Autodesk Inventor part; units mm, degrees
ref_plane "YZ Plane" through (0, 0, 0) normal (1, 0, 0) x (0, 1, 0)
ref_plane "XZ Plane" through (0, 0, 0) normal (0, 1, 0) x (-1, 0, 0)
ref_plane "XY Plane" through (0, 0, 0) normal (0, 0, 1) x (1, 0, 0)
sketch "スケッチ1" plane through (0, 0, 0) normal (0, 0, 1) x (1, 0, 0)
  line L0 (0, 0) -> (122, 0)
  line L1 (122, 0) -> (122, 22)
  line L2 (122, 22) -> (0, 22)
  line L3 (0, 22) -> (0, 0)
  dimension "d0" = 122
  dimension "d1" = 22
extrude "押し出し1" add sketch "スケッチ1" along normal blind 2
fillet "フィレット1" radius 2 4 edges at (122, 22, 1) (122, 0, 1) (0, 22, 1) (0, 0, 1)
sketch "スケッチ2" plane through (0, 0, 2) normal (0, 0, 1) x (1, 0, 0)
  line L0 (0, 4.5) -> (122, 4.5)
  line L1 (122, 2) -> (122, 20)
  line L2 (2, 0) -> (120, 0)
  line L3 (0, 20) -> (0, 2)
  point P0 (0, 0)
  point P1 (11, 4.5)
  point P2 (31, 4.5)
  point P3 (51, 4.5)
  point P4 (61, 4.5)
  point P5 (71, 4.5)
  point P6 (91, 4.5)
  point P7 (111, 4.5)
  dimension "d5" = 4.5
  dimension "d6" = 11
  dimension "d7" = 11
  dimension "d8" = 20
  dimension "d9" = 20
  dimension "d10" = 10
  dimension "d11" = 10
  dimension "d12" = 20
hole "穴1" at (11, 4.5, 2) at (31, 4.5, 2) at (51, 4.5, 2) at (61, 4.5, 2) at (71, 4.5, 2) at (91, 4.5, 2) at (111, 4.5, 2) direction (0, 0, -1) diameter 3.2 end through all
properties part number "line_sensor" material "アセタール樹脂、黒"
Read the model definition and answer for the solid it produces. Units are mm, in the model's axes. Round coordinates to 2 decimals unless told otherwise and drop trailing zeros. Write each loop counter-clockwise with the first axis right and the second up, starting at its lowest first coordinate (ties: lowest second). Pieces come first, ordered by that corner, then holes.
Q1. A straight line is drawn through the part: line 1 (Y direction, x = 51, z = 1.45). Find the intervals that lie inside material, in ascending order.
Values:
line 1: y = 0 to 2.9, 6.1 to 22
Q2. Find section C-C on y = 4.5. State how many separate pieces and enclosed holes the cut face has, and give its area (3 significant figures).
Values:
separate pieces: 8
enclosed holes: 0
area: 199 mm2
Q3. The mould has two halves that part along X. Classify faces 1 (the face through (0, 11, 1)), 2 (the face through (121.4, 0.57, 1.01)), 3 (the face through (89.414, 4.708, 0.986)), 4 (the face through (60, 0, 1)): released by +X, released by -X, zero draft, split by the parting line, or undercut.
Values:
face 1: released by -X
face 2: released by +X
face 3: undercut
face 4: zero draft
Q4. Find section B-B on z = 1.3. Determine the outline of the cut face in (x, y).
Values:
outline: (0, 2) arc R2 ccw to (2, 0) - (120, 0) arc R2 ccw to (122, 2) - (122, 20) arc R2 ccw to (120, 22) - (2, 22) arc R2 ccw to (0, 20) - close; hole circle Ø3.2 at (11, 4.5); hole circle Ø3.2 at (31, 4.5); hole circle Ø3.2 at (51, 4.5); hole circle Ø3.2 at (61, 4.5); hole circle Ø3.2 at (71, 4.5); hole circle Ø3.2 at (91, 4.5); hole circle Ø3.2 at (111, 4.5)
Q5. Find section A-A on x = 51. Determine the outline of the cut face in (y, z).
Values:
outline: (0, 0) - (2.9, 0) - (2.9, 2) - (0, 2) - close; (6.1, 0) - (22, 0) - (22, 2) - (6.1, 2) - close
